Design review of the part shown in the three views and the two pictorial views. Dimensions are in mm from the part's minimum x, y and z. A direction names the side the tool comes from. Coordinates: 2 decimals unless noted, no trailing zeros. Use CSV: the item, a comma, the result in double quotes.
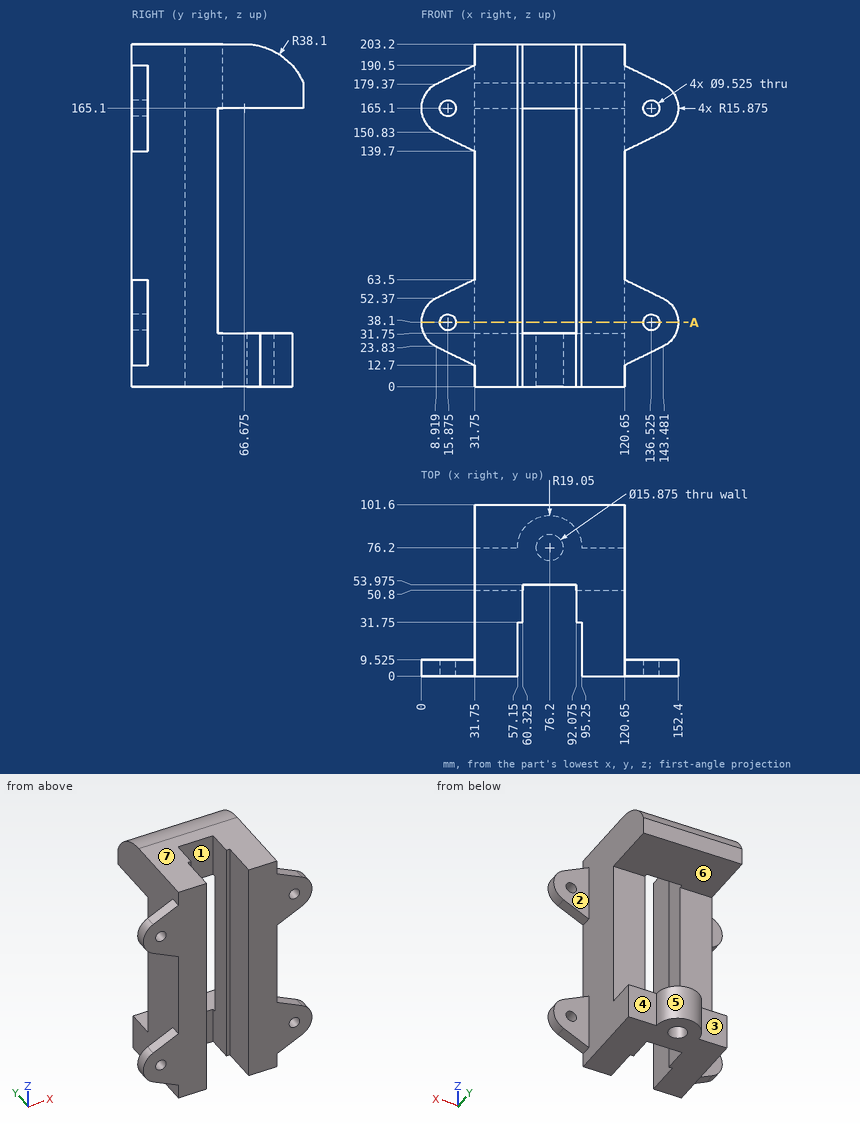
(1) For the marked faces 1, 2, 3 and 4, list the 3-axis set-ups (+Z, -Z, +X, -X, +Y, -Y) from which the entire face can be reached by the end or side of a thin tool; tool diameter is ignored.
The answers:
face 1,"+Z, -Z, -Y"
face 2,"+Z, -Z, +X, +Y"
face 3,"-Z, -X, +Y"
face 4,"-Z, +X, +Y"
(2) Wall thickness on probe 1 along X at (y, z) = (5.25, 38.1); probe 2 along X at (y, z) = (29.5, 44); probe 3 along Z at (x, y) = (81, 61.5): over which ranges is each line inside the solid? List them lowest first.
The answers:
probe 1,"x = 0 to 11.11, 20.64 to 57.15, 95.25 to 131.76, 141.29 to 152.4"
probe 2,"x = 31.75 to 57.15, 95.25 to 120.65"
probe 3,"z = 0 to 31.75, 165.1 to 203.2"
(3) The part is to be moulded in two halves that separate along Z. For the marked faces 5, 6 and 7, say which applies: pulls with the +Z half, pulls with the -Z half, needs draft (parallel to the pull), parting line crosses it, or undercut.
The answers:
face 5,"needs draft"
face 6,"undercut"
face 7,"pulls with the +Z half"
(4) Add section A-A on z = 38.1. Give the number of separate pieces and of enclosed holes in the cut face, and give its area (4 significant figures).
The answers:
separate pieces,"4"
enclosed holes,"0"
area,"3,125 mm2"
(5) Clearance check with flat-ended pins moving along their axes: P1, Ø16, axis at x = 18, z = 166, coming from the +Y side (3 decimals); P2, Ø6.5, axis at y = 44.5, z = 73.5, coming from the +X side; P3, Ø18, axis at y = 44, z = 101.5, coming from the -X side. State where each tip first meets the part, or that it passes through.
The answers:
P1,"stops at y = 9.525"
P2,"stops at x = 120.65"
P3,"stops at x = 31.75"
